For this review, take the finished solid that the model builds, in its own axes (mm). Face numbers are marked on the shaded views. Give positions to 0.01 mm unless a question says otherwise; leave off trailing zeros. Loops run counter-clockwise (first coordinate to the right, second up) from the corner with the lowest first, then second, coordinate; pieces in that order, holes last. Notation, with made-up numbers: (5, 68) - (45, 68) arc R21 ccw to (45, 77) - close; hole circle Ø8 at (85, 32). An arc over 180 degrees is marked (long way). Put each result on its own line as item: value. Start each with the question number.
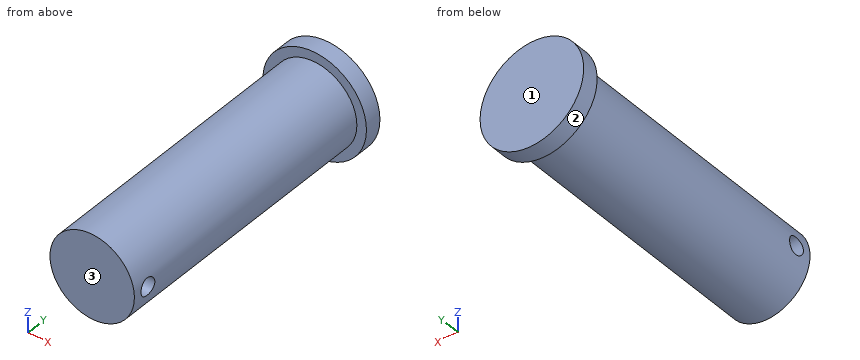
from build123d import *

# Parameters (mm, degrees)
F0_R     = 6.135
F1_DEPTH = 2
F2_R     = 5
F3_DEPTH = 33
F5_R     = 1.024989
F6_DEPTH = 11.136


with BuildPart() as f1:
    # F0 (on Front) → F1 (new body)
    with BuildSketch(Plane.XZ):
        Circle(F0_R)
    extrude(amount=F1_DEPTH)

    # F2 (on face) → F3 (join)
    with BuildSketch(Plane.XZ.offset(2)):
        Circle(F2_R)
    extrude(amount=F3_DEPTH)

    # F5 (on offset) → F6 (cut, through all)
    with BuildSketch(Plane.YZ.offset(5)):
        with Locations((-32.996107, 0)):
            Circle(F5_R)
    extrude(amount=-F6_DEPTH, mode=Mode.SUBTRACT)


solid = f1.part
1) Take a section at D-D on z = 4.25. State the section outline as (x, y) points, and give its area (3 significant figures).
2) Take a section at C-C on y = -14. State the section outline as (x, z) points.
3) Mouldability with a two-part tool opening along Y and no side actions: class the marked faces 1, 2 and 3 as released by +Y, released by -Y, zero draft, split by the parting line, or undercut.
4) Take a section at B-B on z = 0. State the section outline as (x, y) points (3 decimals).
5) Take a section at A-A on x = 0. State the section outline as (y, z) points (3 decimals).
6) Insertion check: P1, Ø4, axis at x = -0.5, y = -30, coming from the -Z side; P2, Ø2, axis at x = -4, z = -5, coming from the +Y side; P3, Ø2.5, axis at y = -33, z = 0, coming from the +X side. Each pin has a flat end and moves straight along its axis. Give the tip position at first contact, or say it passes through.
7) Wall thickness on probe 1 along Y at (x, z) = (2.5, 0); probe 2 along X at (y, z) = (-28.5, -0.25); probe 3 along Y at (x, z) = (5, -2.75): over which ranges is each line inside the solid? List them lowest first.
Answers follow:
1. outline: (-4.42, -2) - (-2.63, -2) - (-2.63, -35) - (2.63, -35) - (2.63, -2) - (4.42, -2) - (4.42, 0) - (-4.42, 0) - close
1. area: 192 mm2
2. outline: circle Ø10 at (0, 0)
3. face 1: released by +Y
3. face 2: zero draft
3. face 3: released by -Y
4. outline: (-6.135, -2) - (-5, -2) - (-5, -31.971) - (5, -31.971) - (5, -2) - (6.135, -2) - (6.135, 0) - (-6.135, 0) - close; (-5, -35) - (5, -35) - (5, -34.021) - (-5, -34.021) - close
5. outline: (-35, -5) - (-2, -5) - (-2, -6.135) - (0, -6.135) - (0, 6.135) - (-2, 6.135) - (-2, 5) - (-35, 5) - close; hole circle Ø2.05 at (-32.996, 0)
6. P1: z = -5
6. P2: y = 0
6. P3: x = 5
7. probe 1: -35 to -34.02, -31.97 to 0
7. probe 2: -4.99 to 4.99
7. probe 3: -2 to 0
